Source: CAD feature listing. Evaluate the final solid. Frame: model axes, mm. Face numbers are marked on the shaded views. A direction names the side the tool comes from. Coordinates: 2 decimals unless noted, no trailing zeros. Write each loop counter-clockwise with the first axis right and the second up, starting at its lowest first coordinate (ties: lowest second). Pieces come first, ordered by that corner, then holes. Notation, with made-up numbers: (-37, 59.25) -> (12, 59.25) arc R22 cw to (12, 98.25) -> close; hole circle Ø5 at (-18.5, -14.75). An arc over 180 degrees is marked (long way). One line per item, written item: value. Start each with the question number.
1. Section query D-D, the plane z = -4.25. Output: boundary loops of the cut face in (x, y).
2. First-contact query: P1, Ø1, axis at x = -12, y = 7, coming from the -Z side; P2, Ø5.5, axis at x = -12.7, z = 0, coming from the -Y side; P3, Ø1, axis at y = 9.5, z = 1, coming from the +X side; P4, Ø4, axis at x = 13, z = -1, coming from the +Y side. Flat tips, straight axial feed; report the tip coordinate or a pass-through.
3. Section query B-B, the plane x = 12.7. Output: boundary loops of the cut face in (y, z), and give its area (3 significant figures).
4. Mould query, pull axis X, two halves, no side actions, for the marked faces 4, 5, 6 and 7. Classes: released by +X, released by -X, zero draft, split by the parting line, or undercut.
5. Access query for the marked faces 1, 2 and 3. Directions: +Z, -Z, +X, -X, +Y, -Y. A direction counts if a zero-diameter tool reaches every point of the face in a straight line with its end or side. Return the directions, or none.
6. Section query C-C, the plane y = 3. Output: boundary loops of the cut face in (x, z), and give its area (3 significant figures).
7. Section query A-A, the plane z = 0. Output: boundary loops of the cut face in (x, y).
8. Line query: line 1 (X direction, y = 3.75, z = 0); line 2 (Y direction, x = 0, z = 2.75); line 3 (X direction, y = 5.5, z = -0.5). Output: solid intervals per line, ascending.
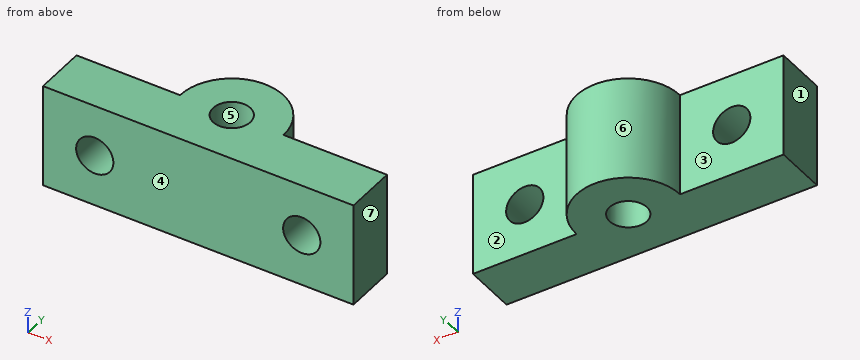
from build123d import *

# Parameters (mm, degrees)
SKETCH1_W           = 38.1
SKETCH1_H           = 12.7
SKETCH1_R           = 2.286
BOSS_EXTRUDE1_DEPTH = 6.35
SKETCH4_R           = 6.35
BOSS_EXTRUDE2_DEPTH = 12.7
SKETCH2_R           = 2.286
CUT_EXTRUDE1_DEPTH  = 27.181720723


with BuildPart() as part:
    # Sketch1 → Boss-Extrude1 (new body)
    with BuildSketch(Plane(origin=(0, 0, 0), x_dir=(1, 0, 0), z_dir=(0, 1, 0))):
        Rectangle(SKETCH1_W, SKETCH1_H)
        with Locations(Location((-12.7, 0, 0), (0, 0, 270))):
            Circle(SKETCH1_R, mode=Mode.SUBTRACT)
        with Locations(Location((12.7, 0, 0), (0, 0, 270))):
            Circle(SKETCH1_R, mode=Mode.SUBTRACT)
    extrude(amount=BOSS_EXTRUDE1_DEPTH)

    # Sketch4 → Boss-Extrude2 (add)
    with BuildSketch(Plane.XY.offset(6.35)):
        with Locations((0, 6.35)):
            Circle(SKETCH4_R)
    extrude(amount=-BOSS_EXTRUDE2_DEPTH)

    # Sketch2 → Cut-Extrude1 (cut, through all)
    with BuildSketch(Plane.XY.offset(6.35)):
        with Locations((0, 6.35)):
            Circle(SKETCH2_R)
    extrude(amount=-CUT_EXTRUDE1_DEPTH, mode=Mode.SUBTRACT)


solid = part.part
Computed values:
1. outline: (-19.05, 0) -> (19.05, 0) -> (19.05, 6.35) -> (6.35, 6.35) arc R6.35 ccw to (-6.35, 6.35) -> (-19.05, 6.35) -> close; hole circle Ø4.57 at (0, 6.35)
2. P1: passes through
2. P2: stops at y = 0
2. P3: stops at x = 5.77
2. P4: stops at y = 6.35
3. outline: (0, -6.35) -> (6.35, -6.35) -> (6.35, -2.29) -> (0, -2.29) -> close; (0, 2.29) -> (6.35, 2.29) -> (6.35, 6.35) -> (0, 6.35) -> close
3. area: 51.6 mm²
4. face 4: zero draft
4. face 5: undercut
4. face 6: split by the parting line
4. face 7: released by +X
5. face 1: +Z, -Z, -X, +Y, -Y
5. face 2: +Z, -Z, +X, +Y
5. face 3: +Z, -Z, -X, +Y
6. outline: (-19.05, -6.35) -> (19.05, -6.35) -> (19.05, 6.35) -> (-19.05, 6.35) -> close; hole circle Ø4.57 at (-12.7, 0); hole circle Ø4.57 at (12.7, 0)
6. area: 451 mm²
7. outline: (-19.05, 0) -> (-14.99, 0) -> (-14.99, 6.35) -> (-19.05, 6.35) -> close; (-10.41, 0) -> (10.41, 0) -> (10.41, 6.35) -> (6.35, 6.35) arc R6.35 ccw to (-6.35, 6.35) -> (-10.41, 6.35) -> close; (14.99, 0) -> (19.05, 0) -> (19.05, 6.35) -> (14.99, 6.35) -> close; hole circle Ø4.57 at (0, 6.35)
8. line 1: x = -19.05 to -14.99, -10.41 to 10.41, 14.99 to 19.05
8. line 2: y = 0 to 4.06, 8.64 to 12.7
8. line 3: x = -19.05 to -14.93, -10.47 to -2.12, 2.12 to 10.47, 14.93 to 19.05
